from build123d import *

# Parameters (mm, degrees)
SKETCH1_R           = 5
BOSS_EXTRUDE1_DEPTH = 126
CUT_EXTRUDE1_DEPTH  = 8
CUT_EXTRUDE2_START  = -8
CUT_EXTRUDE2_DEPTH  = 8


with BuildPart() as part:
    # Sketch1 → Boss-Extrude1 (new body)
    with BuildSketch(Plane(origin=(0, 0, 0), x_dir=(0, 0, -1), z_dir=(1, 0, 0))):
        Circle(SKETCH1_R)
    extrude(amount=BOSS_EXTRUDE1_DEPTH)

    # Sketch2 → Cut-Extrude1 (cut)
    with BuildSketch(Plane(origin=(126, 0, 0), x_dir=(0, 0, -1), z_dir=(1, 0, 0))):
        with BuildLine():
            Line((-2.688276978, -1.019211407), (0.225725397, -2.866125092))
            ThreePointArc((0.225725397, -2.866125092), (2.428335312, -1.539094738), (2.688276978, 1.019211407))
            Line((2.688276978, 1.019211407), (-0.225725397, 2.866125092))
            ThreePointArc((-0.225725397, 2.866125092), (-2.428335312, 1.539094738), (-2.688276978, -1.019211407))
        make_face()
    extrude(amount=-CUT_EXTRUDE1_DEPTH, mode=Mode.SUBTRACT)

    # Sketch3 → Cut-Extrude2 (cut)
    with BuildSketch(Plane.ZY.offset(CUT_EXTRUDE2_START)):
        with BuildLine():
            Line((0.225725397, 2.866125092), (-2.688276978, 1.019211407))
            ThreePointArc((-2.688276978, 1.019211407), (-2.428335312, -1.539094738), (-0.225725397, -2.866125092))
            Line((-0.225725397, -2.866125092), (2.688276978, -1.019211407))
            ThreePointArc((2.688276978, -1.019211407), (2.428335312, 1.539094738), (0.225725397, 2.866125092))
        make_face()
    extrude(amount=CUT_EXTRUDE2_DEPTH, mode=Mode.SUBTRACT)


solid = part.part
Could you check a few things on this model? Use its own coordinates, in mm. A direction names the side the tool comes from. Round coordinates to 2 decimals unless told otherwise and drop trailing zeros. Write each loop counter-clockwise with the first axis right and the second up, starting at its lowest first coordinate (ties: lowest second). Pieces come first, ordered by that corner, then holes. Notation, with made-up numbers: (-23, 79.5) - (-8, 79.5) arc R25 ccw to (-8, 96.5) - close; hole circle Ø2 at (48, 55.25). An arc over 180 degrees is marked (long way). Put each result on its own line as item: value. Start each with the question number.
(1) Thinking about a two-plate mould opening in Y: for faces 1 (the cylindrical face through (4.056, -1.507, -2.448)), 2 (the flat face through (0, -2.2, 1.2)), 3 (the cylindrical face through (62.12, -4.88, 1.08)), which applies, released by +Y, released by -Y, zero draft, split by the parting line, or undercut?
(2) Will this pin go through, and if not, where does the flat tip stop? pin 1 (2 mm diameter, centred on x = 97, z = 1.5, fed in from +Y).
(3) I need wall thicknesses on probe 1 along X at (y, z) = (1, 1.25); probe 2 along Y at (x, z) = (21.5, 0.25); probe 3 along Y at (x, z) = (113, -3). Which ranges of each line are inside material? Lowest first, please.
(4) I want a section at B-B, the plane x = 71.5. Please give me the cut outline in (y, z).
(5) For faces 4 (the flat face through (126, -2.2, 1.2)), 5 (the flat face through (122.1, -1.9, 1.3)), 6 (the flat face through (4.056, 1.956, -1.211)), which set-ups out of +Z, -Z, +X, -X, +Y, -Y let a thin tool reach every point of the face, with its end or its side?
(6) I want a section at A-A, the plane y = 0. Please give me the cut outline in (x, z) (3 decimals).
Here are the results:
1. face 1: undercut
1. face 2: zero draft
1. face 3: split by the parting line
2. pin 1: stops at y = 4.97
3. probe 1: x = 8 to 118
3. probe 2: y = -4.99 to 4.99
3. probe 3: y = -4 to 4
4. outline: circle Ø10 at (0, 0)
5. face 4: +Z, -Z, +X, +Y, -Y
5. face 5: +X
5. face 6: -X
6. outline: (0, -5) - (126, -5) - (126, -2.875) - (118, -2.875) - (118, 2.875) - (126, 2.875) - (126, 5) - (0, 5) - (0, 2.875) - (8, 2.875) - (8, -2.875) - (0, -2.875) - close
